```python
from build123d import *

# Parameters (mm, degrees)
SKETCH1_R           = 1
BOSS_EXTRUDE1_DEPTH = 1.1


with BuildPart() as part:
    # Sketch1 → Boss-Extrude1 (new body)
    # profile 1 of 3: a face of its own
    with BuildSketch(Plane.XY):
        Polygon((-8.343354955, 9.9), (-9.9, 8.343354955), (-9.9, 2.2), (-9.9, -2.2), (-9.9, -8.343354955), (-8.343354955, -9.9), (8.343354955, -9.9), (9.9, -8.343354955), (9.9, -2.2), (9.9, 2.2), (9.9, 8.343354955), (8.343354955, 9.9), align=None)
        Polygon((-8.7, -7.84629868), (-8.7, 7.84629868), (-7.84629868, 8.7), (7.84629868, 8.7), (8.7, 7.84629868), (8.7, -7.84629868), (7.84629868, -8.7), (-7.84629868, -8.7), align=None, mode=Mode.SUBTRACT)
    # profile 2 of 3: a face of its own
    with BuildSketch(Plane.XY):
        with BuildLine():
            Line((-9.9, -2.2), (-9.9, 2.2))
            Line((-9.9, 2.2), (-11.000000224, 2.2))
            ThreePointArc((-11.000000224, 2.2), (-13.200000224, 0), (-11.000000224, -2.2))
            Line((-11.000000224, -2.2), (-9.9, -2.2))
        make_face()
        with Locations((-11.000000224, 0)):
            Circle(SKETCH1_R, mode=Mode.SUBTRACT)
    # profile 3 of 3: a face of its own
    with BuildSketch(Plane.XY):
        with BuildLine():
            Line((11, 2.2), (9.9, 2.2))
            Line((9.9, 2.2), (9.9, -2.2))
            Line((9.9, -2.2), (11, -2.2))
            ThreePointArc((11, -2.2), (13.2, 0), (11, 2.2))
        make_face()
        with Locations((11, 0)):
            Circle(SKETCH1_R, mode=Mode.SUBTRACT)
    extrude(amount=BOSS_EXTRUDE1_DEPTH)


solid = part.part
```
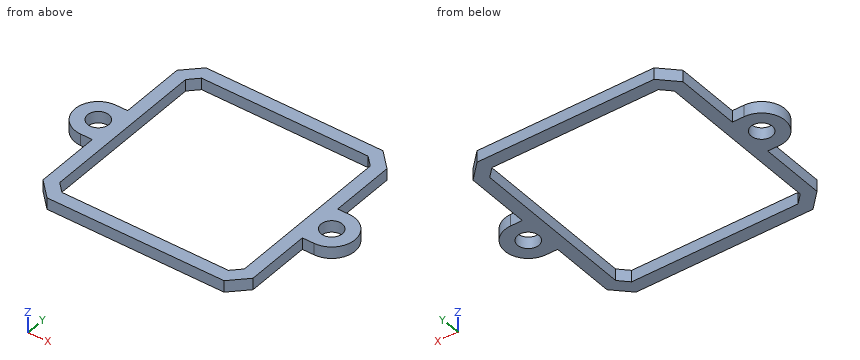
Geometry check sheet. Reference: the model listing, model coordinates, mm. Round coordinates to 2 decimals unless told otherwise and drop trailing zeros. Loops run counter-clockwise (first coordinate to the right, second up) from the corner with the lowest first, then second, coordinate; pieces in that order, holes last. Notation, with made-up numbers: (-17.75, 46.25) - (23.25, 46.25) arc R28 cw to (23.25, 84.25) - close; hole circle Ø11 at (-1.5, 86.5). An arc over 180 degrees is marked (long way). Use a Markdown table: item, result.
Q1. Cross-section at A-A on x = -6.5. Record the cut outline in (y, z), plus the area to 3 significant figures.
Solutions:
| item | result |
|---|---|
| outline | (-9.9, 0) - (-8.7, 0) - (-8.7, 1.1) - (-9.9, 1.1) - close; (8.7, 0) - (9.9, 0) - (9.9, 1.1) - (8.7, 1.1) - close |
| area | 2.64 mm2 |
Q2. Cross-section at C-C on y = 0. Record the cut outline in (x, z).
Solutions:
| item | result |
|---|---|
| outline | (-13.2, 0) - (-12, 0) - (-12, 1.1) - (-13.2, 1.1) - close; (-10, 0) - (-8.7, 0) - (-8.7, 1.1) - (-10, 1.1) - close; (8.7, 0) - (10, 0) - (10, 1.1) - (8.7, 1.1) - close; (12, 0) - (13.2, 0) - (13.2, 1.1) - (12, 1.1) - close |
Q3. Go/stop test with flat-tipped pins: P1, Ø0.6, axis at x = -10.5, z = 0.5, coming from the +Y side; P2, Ø0.6, axis at y = -4, z = 1, coming from the -X side; P3, Ø0.6, axis at x = -10.5, z = 0.5, coming from the -Y side. Record where each tip stops, or that it passes through.
Solutions:
| item | result |
|---|---|
| P1 | stops at y = 2.2 |
| P2 | stops at x = -9.9 |
| P3 | stops at y = -2.2 |
Q4. Material ranges on line 1 (Y direction, x = -5.5, z = 0.35); line 2 (Y direction, x = -10.5, z = 0.35), recorded low to high.
Solutions:
| item | result |
|---|---|
| line 1 | y = -9.9 to -8.7, 8.7 to 9.9 |
| line 2 | y = -2.2 to -0.87, 0.87 to 2.2 |
Q5. Cross-section at B-B on z = 0.65. Record the cut outline in (x, y), plus the area to 3 significant figures.
Solutions:
| item | result |
|---|---|
| outline | (-11, -2.2) - (-9.9, -2.2) - (-9.9, -8.34) - (-8.34, -9.9) - (8.34, -9.9) - (9.9, -8.34) - (9.9, -2.2) - (11, -2.2) arc R2.2 ccw to (11, 2.2) - (9.9, 2.2) - (9.9, 8.34) - (8.34, 9.9) - (-8.34, 9.9) - (-9.9, 8.34) - (-9.9, 2.2) - (-11, 2.2) arc R2.2 ccw to start; hole circle Ø2 at (-11, 0); hole (-8.7, -7.85) - (-7.85, -8.7) - (7.85, -8.7) - (8.7, -7.85) - (8.7, 7.85) - (7.85, 8.7) - (-7.85, 8.7) - (-8.7, 7.85) - close; hole circle Ø2 at (11, 0) |
| area | 104 mm2 |
